from build123d import *

# Parameters (mm, degrees)
TORUS_R        = 7
CYLINDER_R     = 55
CYLINDER_DEPTH = 20


with BuildPart() as torus:
    # Torus → Torus (revolve)
    with BuildSketch(Plane(origin=(0, 0, -18), x_dir=(1, 0, 0), z_dir=(0, -1, 0))):
        with Locations((35, 0)):
            Circle(TORUS_R)
    revolve(axis=Axis((0, 0, -18), (0, 0, 1)))


with BuildPart() as cut001:
    # Cylinder → Cylinder (new body)
    with BuildSketch(Plane.XY.offset(-16)):
        Circle(CYLINDER_R)
    extrude(amount=CYLINDER_DEPTH)

    # Cut001: cut Torus
    add(torus.part, mode=Mode.SUBTRACT)


solid = cut001.part
Input: part model. Units: mm. Frame: model coordinates. Coordinates: 2 decimals unless noted, no trailing zeros. Loops run counter-clockwise (first coordinate to the right, second up) from the corner with the lowest first, then second, coordinate; pieces in that order, holes last. Notation, with made-up numbers: (28, -38) - (45, -38) arc R8 cw to (45, -31) - close; hole circle Ø6 at (61.25, 56). An arc over 180 degrees is marked (long way). Answer in a Markdown table with one row per item. Add a question column.
Item 1: Line query: line 1 along Y through (x, z) = (-8, -13); line 2 along Y through (x, z) = (36, -14); line 3 along Z through (x, y) = (-26, -23.5). Output: solid intervals per line, ascending. Write a range as [from, to].
Item 2: Contact query for flat-ended pins moving along their axis: P1, Ø3, axis at y = 31.5, z = 0, coming from the +X side; P2, Ø3, axis at x = -19, z = -4, coming from the -Y side; P3, Ø3, axis at x = 9.5, z = -2.5, coming from the -Y side. Output: stop coordinate, or through.
Item 3: Section query C-C on z = -3. Return the cut outline in (x, y), then the cut area to 3 significant figures.
Item 4: Section query A-A on y = 0. Return the cut outline in (x, z).
Recorded:
| question | item | result |
|---|---|---|
| 1 | line 1 | [-54.42, -39.09], [-29.02, 29.02], [39.09, 54.42] |
| 1 | line 2 | [-41.58, -19.08], [19.08, 41.58] |
| 1 | line 3 | [-11, 4] |
| 2 | P1 | x = 46.1 |
| 2 | P2 | y = -52.14 |
| 2 | P3 | y = -54.42 |
| 3 | outline | circle Ø110 at (0, 0) |
| 3 | area | 9,500 mm^2 |
| 4 | outline | (-55, -16) - (-41.71, -16) arc R7 cw to (-28.29, -16) - (28.29, -16) arc R7 cw to (41.71, -16) - (55, -16) - (55, 4) - (-55, 4) - close |
